```python
from build123d import *

# Parameters (mm, degrees)
SKETCH1_W           = 37
SKETCH1_H           = 37
SKETCH1_R           = 2.5
SKETCH1_R_2         = 3.175
BOSS_EXTRUDE1_DEPTH = 12.7
SKETCH2_R           = 6.5
SKETCH2_R_2         = 2.5
BOSS_EXTRUDE2_DEPTH = 12.7
FILLET1_R           = 5
CHAMFER1_SIZE       = 1.5


with BuildPart() as part:
    # Sketch1 → Boss-Extrude1 (new body)
    with BuildSketch(Plane(origin=(0, 0, 0), x_dir=(1, 0, 0), z_dir=(0, 1, 0))):
        Rectangle(SKETCH1_W, SKETCH1_H)
        Circle(SKETCH1_R, mode=Mode.SUBTRACT)
        with Locations((-12.7, -12.7)):
            Circle(SKETCH1_R_2, mode=Mode.SUBTRACT)
        with Locations((12.7, -12.7)):
            Circle(SKETCH1_R_2, mode=Mode.SUBTRACT)
        with Locations((12.7, 12.7)):
            Circle(SKETCH1_R_2, mode=Mode.SUBTRACT)
        with Locations((-12.7, 12.7)):
            Circle(SKETCH1_R_2, mode=Mode.SUBTRACT)
    extrude(amount=BOSS_EXTRUDE1_DEPTH)

    # Sketch2 → Boss-Extrude2 (add)
    with BuildSketch(Plane(origin=(0, 12.7, 0), x_dir=(1, 0, 0), z_dir=(0, 1, 0))):
        Circle(SKETCH2_R)
        Circle(SKETCH2_R_2, mode=Mode.SUBTRACT)
    extrude(amount=BOSS_EXTRUDE2_DEPTH)

    # Fillet1
    fillet1_edges = [part.edges().sort_by_distance(p)[0] for p in [
        (-6.5, 12.7, 0),
        (18.5, 6.35, 18.5),
        (-18.5, 6.35, 18.5),
        (-18.5, 6.35, -18.5),
        (18.5, 6.35, -18.5),
    ]]
    fillet(fillet1_edges, radius=FILLET1_R)

    # Chamfer1
    chamfer1_edges = [part.edges().sort_by_distance(p)[0] for p in [
        (-2.5, 25.4, 0),
    ]]
    chamfer(chamfer1_edges, length=CHAMFER1_SIZE)


solid = part.part
```
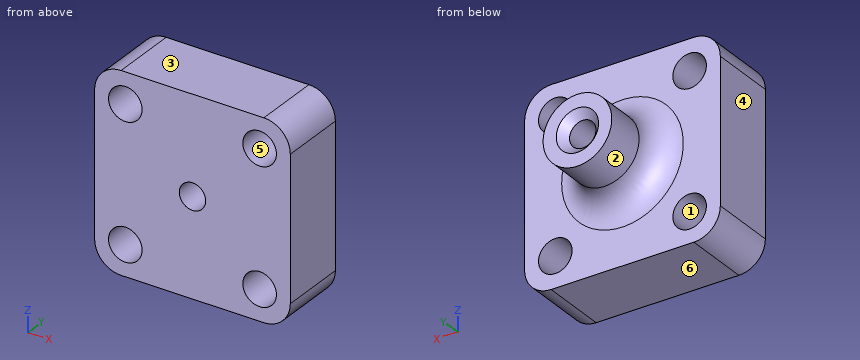
The listing builds one solid part. Answer for the finished solid, in the listing's coordinates (mm). Face numbers are marked on the shaded views. A direction names the side the tool comes from. Coordinates: 2 decimals unless noted, no trailing zeros. Loops run counter-clockwise (first coordinate to the right, second up) from the corner with the lowest first, then second, coordinate; pieces in that order, holes last. Notation, with made-up numbers: (27.25, 19) -> (79.25, 19) arc R20 ccw to (79.25, 34) -> close; hole circle Ø4 at (60, -5.5). An arc over 180 degrees is marked (long way). Return JSON: item names as keys, results as strings. Group by question number.
(1) Given pin 1 Ø10 at (x, z) = (12.7, 12.7) entering from +Y; pin 2 Ø1 at (x, y) = (-4.5, 20) entering from -Z; pin 3 Ø6 at (x, y) = (-3.5, 17.5) entering from +Z, each flat-ended and moving along its own axis, determine where each tip first touches the part or whether it passes through.
(2) Determine the mould class of the marked faces 3, 4, 5 and 6 for opening direction Z: released by +Z, released by -Z, zero draft, split by the parting line, or undercut.
(3) A cutting plane is placed at C-C on x = 12.7. Write down the section's boundary in (y, z) (3 decimals), and give its area (3 significant figures).
(4) A cutting plane is placed at D-D on y = 2.25. Write down the section's boundary in (x, z) (3 decimals).
(5) A cutting plane is placed at A-A on z = 0. Write down the section's boundary in (x, y).
(6) Which of the six approach directions +Z, -Z, +X, -X, +Y, -Y give full straight-line access (tool end or side, diameter ignored) to the marked faces 1 and 2?
(7) Find the intervals of material crossed by probe 1 along Z at (x, y) = (-12.7, 4.25) (3 decimals); probe 2 along X at (y, z) = (9.5, 0), in increasing order. Write a range as from..to.
(8) A cutting plane is placed at B-B on x = 0. Write down the section's boundary in (y, z), and give its area (3 significant figures).
The answers:
{
 "1": {"pin 1": "stops at y = 12.7", "pin 2": "stops at z = -5.12", "pin 3": "stops at z = 7.1"},
 "2": {"face 3": "released by +Z", "face 4": "zero draft", "face 5": "undercut", "face 6": "released by -Z"},
 "3": {"outline": "(0, -18.5) -> (12.7, -18.5) -> (12.7, -15.875) -> (0, -15.875) -> close; (0, -9.525) -> (12.7, -9.525) -> (12.7, 9.525) -> (0, 9.525) -> close; (0, 15.875) -> (12.7, 15.875) -> (12.7, 18.5) -> (0, 18.5) -> close", "area": "309 mm^2"},
 "4": {"outline": "(-18.5, -13.5) arc R5 ccw to (-13.5, -18.5) -> (13.5, -18.5) arc R5 ccw to (18.5, -13.5) -> (18.5, 13.5) arc R5 ccw to (13.5, 18.5) -> (-13.5, 18.5) arc R5 ccw to (-18.5, 13.5) -> close; hole circle Ø6.35 at (-12.7, -12.7); hole circle Ø6.35 at (-12.7, 12.7); hole circle Ø5 at (0, 0); hole circle Ø6.35 at (12.7, -12.7); hole circle Ø6.35 at (12.7, 12.7)"},
 "5": {"outline": "(-18.5, 0) -> (-2.5, 0) -> (-2.5, 23.9) -> (-4, 25.4) -> (-6.5, 25.4) -> (-6.5, 17.7) arc R5 cw to (-11.5, 12.7) -> (-18.5, 12.7) -> close; (2.5, 0) -> (18.5, 0) -> (18.5, 12.7) -> (11.5, 12.7) arc R5 cw to (6.5, 17.7) -> (6.5, 25.4) -> (4, 25.4) -> (2.5, 23.9) -> close"},
 "6": {"face 1": "+Y, -Y", "face 2": "+Y"},
 "7": {"probe 1": "z = -18.5..-15.875, -9.525..9.525, 15.875..18.5", "probe 2": "x = -18.5..-2.5, 2.5..18.5"},
 "8": {"outline": "(0, -18.5) -> (12.7, -18.5) -> (12.7, -11.5) arc R5 cw to (17.7, -6.5) -> (25.4, -6.5) -> (25.4, -4) -> (23.9, -2.5) -> (0, -2.5) -> close; (0, 2.5) -> (23.9, 2.5) -> (25.4, 4) -> (25.4, 6.5) -> (17.7, 6.5) arc R5 cw to (12.7, 11.5) -> (12.7, 18.5) -> (0, 18.5) -> close", "area": "516 mm^2"}
}
